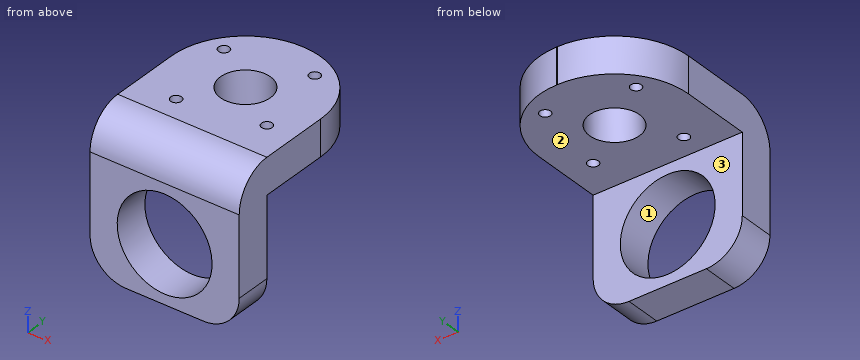
from build123d import *

# Parameters (mm, degrees)
BOSS_EXTRUDE1_DEPTH = 5
BOSS_EXTRUDE2_START = -5
SKETCH2_W           = 20.75
SKETCH2_H           = 5
BOSS_EXTRUDE2_DEPTH = 16
SKETCH3_R           = 6.6
CUT_EXTRUDE1_DEPTH  = 28.634048292
FILLET2_R           = 5
FILLET3_R           = 5
SKETCH5_R           = 3.475
SKETCH5_R_2         = 0.75
CUT_EXTRUDE3_DEPTH  = 27.549776364


with BuildPart() as part:
    # Sketch1 → Boss-Extrude1 (new body)
    with BuildSketch(Plane.XY):
        with BuildLine():
            Line((-0.075, 12.5), (0.075, 12.5))
            ThreePointArc((0.075, 12.5), (7.358199846, 9.483199846), (10.375, 2.2))
            Line((10.375, 2.2), (10.375, -12.5))
            Line((10.375, -12.5), (-10.375, -12.5))
            Line((-10.375, -12.5), (-10.375, 2.2))
            ThreePointArc((-10.375, 2.2), (-7.358199846, 9.483199846), (-0.075, 12.5))
        make_face()
    extrude(amount=BOSS_EXTRUDE1_DEPTH)

    # Sketch2 → Boss-Extrude2 (add)
    with BuildSketch(Plane.XY.offset(5).offset(BOSS_EXTRUDE2_START)):
        with Locations((0, -10)):
            Rectangle(SKETCH2_W, SKETCH2_H)
    extrude(amount=-BOSS_EXTRUDE2_DEPTH)

    # Sketch3 → Cut-Extrude1 (cut, through all)
    with BuildSketch(Plane(origin=(0, -7.5, 0), x_dir=(1, 0, 0), z_dir=(0, 1, 0))):
        with Locations(Location((0, 8, 0), (0, 0, 270))):
            Circle(SKETCH3_R)
    extrude(amount=-CUT_EXTRUDE1_DEPTH, mode=Mode.SUBTRACT)

    # Fillet2
    fillet2_edges = [part.edges().sort_by_distance(p)[0] for p in [
        (10.375, -10, -16),
        (-10.375, -10, -16),
    ]]
    fillet(fillet2_edges, radius=FILLET2_R)

    # Fillet3
    fillet3_edges = [part.edges().sort_by_distance(p)[0] for p in [
        (0, -12.5, 5),
    ]]
    fillet(fillet3_edges, radius=FILLET3_R)

    # Sketch5 → Cut-Extrude3 (cut, through all)
    with BuildSketch(Plane.XY.offset(5)):
        with Locations((-0.075, 2.2)):
            Circle(SKETCH5_R)
        with Locations((-6.613093573, 6.810133667)):
            Circle(SKETCH5_R_2)
        with Locations((4.535133667, 8.738093573)):
            Circle(SKETCH5_R_2)
        with Locations((-4.685133667, -4.338093573)):
            Circle(SKETCH5_R_2)
        with Locations((6.463093573, -2.410133667)):
            Circle(SKETCH5_R_2)
    extrude(amount=-CUT_EXTRUDE3_DEPTH, mode=Mode.SUBTRACT)


solid = part.part
Could you check a few things on this model? Use its own coordinates, in mm. Face numbers are marked on the shaded views. Give positions to 0.01 mm unless a question says otherwise; leave off trailing zeros. Write each loop counter-clockwise with the first axis right and the second up, starting at its lowest first coordinate (ties: lowest second). Pieces come first, ordered by that corner, then holes. Notation, with made-up numbers: (-16.75, 47.5) - (-1.75, 47.5) arc R22 ccw to (-1.75, 82.5) - close; hole circle Ø1 at (28.5, 77). An arc over 180 degrees is marked (long way). Use CSV: the item, a comma, the result in double quotes. Start each with the question number.
Item 1: I want a section at C-C, the plane y = -2.75. Please give me the cut outline in (x, z) (3 decimals), then the cut area to 3 significant figures.
Item 2: I'm going to push flat-ended pins straight in: pin 1 (0.9 mm diameter, centred on x = 6.46, y = -2.41, fed in from +Z); pin 2 (6 mm diameter, centred on x = 2, y = -0.5, fed in from -Z); pin 3 (3 mm diameter, centred on x = -5.5, z = 2, fed in from -Y). Where does each tip first touch, or does it pass through?
Item 3: I want a section at A-A, the plane z = -8. Please give me the cut outline in (x, y) (3 decimals).
Item 4: If I drill on line 1 along X through (y, z) = (-8.95, -8) (3 decimals); line 2 along Z through (x, y) = (-5.75, -6); line 3 along Y through (x, z) = (5, 0.25), over which ranges is the centre line in solid material (lowest first)?
Item 5: If we mould it in two halves opening along Z, with no side actions, what happens to the marked faces 1, 2 and 3? For each: pulls with the +Z half, pulls with the -Z half, needs draft (parallel to the pull), parting line crosses it, or undercut.
Item 6: I want a section at D-D, the plane x = -6.25. Please give me the cut outline in (y, z).
Item 7: I want a section at B-B, the plane x = -2.5. Please give me the cut outline in (y, z), then the cut area to 3 significant figures.
Findings:
1,outline,"(-10.375, 0) - (5.795, 0) - (5.795, 5) - (-10.375, 5) - close; (7.132, 0) - (10.375, 0) - (10.375, 5) - (7.132, 5) - close"
1,area,"97.1 mm2"
2,pin 1,"passes through"
2,pin 2,"stops at z = 0"
2,pin 3,"stops at y = -12.47"
3,outline,"(-10.375, -12.5) - (-6.6, -12.5) - (-6.6, -7.5) - (-10.375, -7.5) - close; (6.6, -12.5) - (10.375, -12.5) - (10.375, -7.5) - (6.6, -7.5) - close"
4,line 1,"x = -10.375 to -6.6, 6.6 to 10.375"
4,line 2,"z = 0 to 5"
4,line 3,"y = -12.49 to 8.15, 9.33 to 11.25"
5,face 1,"undercut"
5,face 2,"pulls with the -Z half"
5,face 3,"needs draft"
6,outline,"(-12.5, -15.92) - (-7.5, -15.92) - (-7.5, -10.12) - (-12.5, -10.12) - close; (-12.5, -5.88) - (-7.5, -5.88) - (-7.5, 0) - (6.15, 0) - (6.15, 5) - (-7.5, 5) arc R5 ccw to (-12.5, 0) - close; (7.47, 0) - (10.44, 0) - (10.44, 5) - (7.47, 5) - close"
7,outline,"(-12.5, -16) - (-7.5, -16) - (-7.5, -14.11) - (-12.5, -14.11) - close; (-12.5, -1.89) - (-7.5, -1.89) - (-7.5, 0) - (-0.29, 0) - (-0.29, 5) - (-7.5, 5) arc R5 ccw to (-12.5, 0) - close; (4.69, 0) - (12.21, 0) - (12.21, 5) - (4.69, 5) - close"
7,area,"112 mm2"
